from build123d import *

# Parameters (mm, degrees)
SKETCH1_W           = 38.1
SKETCH1_H           = 19.05
SKETCH1_R           = 3.175
SKETCH1_H_2         = 12.7
BOSS_EXTRUDE2_DEPTH = 12.7
SKETCH3_W           = 12.7
SKETCH3_H           = 31.75
SKETCH3_H_2         = 12.7
BOSS_EXTRUDE3_DEPTH = 38.1


with BuildPart() as part:
    # Sketch1 → Boss-Extrude2 (new body)
    # profile 1 of 3: a face of its own
    with BuildSketch(Plane(origin=(0, 0, 0), x_dir=(1, 0, 0), z_dir=(0, 1, 0))):
        Rectangle(SKETCH1_W, SKETCH1_H)
        with Locations(Location((0, 0, 0), (0, 0, 270))):
            Circle(SKETCH1_R, mode=Mode.SUBTRACT)
    # profile 2 of 3: a face of its own
    with BuildSketch(Plane(origin=(0, 0, 0), x_dir=(1, 0, 0), z_dir=(0, 1, 0))):
        with Locations((0, -15.875)):
            Rectangle(SKETCH1_W, SKETCH1_H_2)
    # profile 3 of 3: a face of its own
    with BuildSketch(Plane(origin=(0, 0, 0), x_dir=(1, 0, 0), z_dir=(0, 1, 0))):
        with Locations((0, -31.75)):
            Rectangle(SKETCH1_W, SKETCH1_H)
        with Locations(Location((0, -31.75, 0), (0, 0, 270))):
            Circle(SKETCH1_R, mode=Mode.SUBTRACT)
    extrude(amount=BOSS_EXTRUDE2_DEPTH)

    # Sketch3 → Boss-Extrude3 (add)
    with BuildSketch(Plane.XY.offset(34.925)):
        with BuildLine():
            ThreePointArc((-31.75, 31.75), (-38.1, 38.1), (-44.45, 31.75))
            Line((-44.45, 31.75), (-57.15, 31.75))
            ThreePointArc((-57.15, 31.75), (-38.1, 50.8), (-19.05, 31.75))
            Line((-19.05, 31.75), (-31.75, 31.75))
        make_face()
        with Locations((-25.4, 15.875)):
            Rectangle(SKETCH3_W, SKETCH3_H)
        with Locations((-50.8, 25.4)):
            Rectangle(SKETCH3_W, SKETCH3_H_2)
    extrude(amount=-BOSS_EXTRUDE3_DEPTH)


solid = part.part
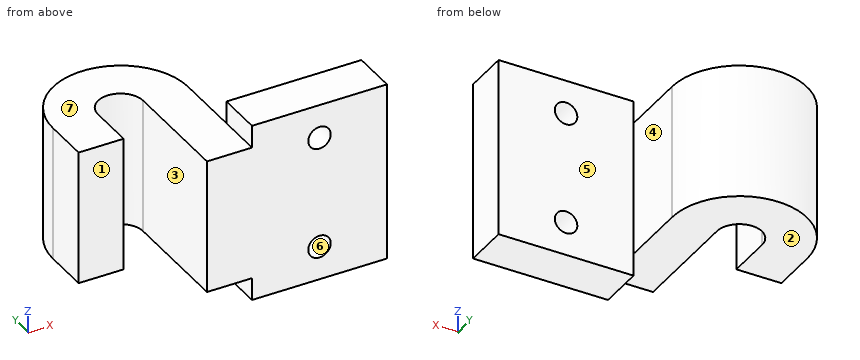
Geometry check sheet. Reference: the model listing, model coordinates, mm. Face numbers are marked on the shaded views. A direction names the side the tool comes from. Round coordinates to 2 decimals unless told otherwise and drop trailing zeros. Loops run counter-clockwise (first coordinate to the right, second up) from the corner with the lowest first, then second, coordinate; pieces in that order, holes last. Notation, with made-up numbers: (82.5, -4.75) - (133.5, -4.75) arc R23 ccw to (133.5, 18.25) - close; hole circle Ø1 at (-26.75, 80). An arc over 180 degrees is marked (long way). One line per question, with ' | ' between items. Start each with the question number.
1. Cross-section at A-A on x = 0. Record the cut outline in (y, z) (3 decimals), then the cut area to 3 significant figures.
2. Cross-section at D-D on y = 11. Record the cut outline in (x, z) (3 decimals), then the cut area to 3 significant figures.
3. Cross-section at B-B on y = 26.5. Record the cut outline in (x, z) (3 decimals), then the cut area to 3 significant figures.
4. Tool access check on the marked faces 1, 2, 3 and 4. Record the directions out of +Z, -Z, +X, -X, +Y, -Y that give a thin tool (end or side, any length) a straight path to the whole face; none if there is none.
5. Cross-section at C-C on z = 0. Record the cut outline in (x, y) (3 decimals).
6. Depth check by flat-ended pin: pin 1 (2 mm diameter, centred on x = 4.5, z = 21, fed in from +Y); pin 2 (6 mm diameter, centred on y = 11, z = -2.5, fed in from -X); pin 3 (8 mm diameter, centred on x = -25, z = 0, fed in from +Y); pin 4 (12 mm diameter, centred on x = 8, z = 30.5, fed in from -Y). Enter the tip coordinate at first touch or a pass-through.
7. Scan lines: line 1 (X direction, y = 28.5, z = 7); line 2 (X direction, y = 3, z = 0) (3 decimals); line 3 (Z direction, x = -21, y = 29.5) (3 decimals). Record each from-to range of solid material in increasing order. Write a range as [from, to].
8. Draft check along Z on the marked faces 5, 6 and 7. Enter one of: released by +Z, released by -Z, zero draft, split by the parting line, or undercut.
Taken from the geometry:
1) outline: (0, -9.525) - (12.7, -9.525) - (12.7, -3.175) - (0, -3.175) - close; (0, 3.175) - (12.7, 3.175) - (12.7, 28.575) - (0, 28.575) - close; (0, 34.925) - (12.7, 34.925) - (12.7, 41.275) - (0, 41.275) - close | area: 484 mm²
2) outline: (-31.75, -3.175) - (-19.05, -3.175) - (-19.05, -9.525) - (19.05, -9.525) - (19.05, 41.275) - (-19.05, 41.275) - (-19.05, 34.925) - (-31.75, 34.925) - close; hole circle Ø6.35 at (0, 0); hole circle Ø6.35 at (0, 31.75) | area: 2,360 mm²
3) outline: (-57.15, -3.175) - (-44.45, -3.175) - (-44.45, 34.925) - (-57.15, 34.925) - close; (-31.75, -3.175) - (-19.05, -3.175) - (-19.05, 34.925) - (-31.75, 34.925) - close | area: 968 mm²
4) face 1: +Z, -Z, -X, -Y | face 2: -Z, -X, +Y, -Y | face 3: +Z, -Z, -Y | face 4: +Z, -Z, +X, +Y
5) outline: (-57.15, 19.05) - (-44.45, 19.05) - (-44.45, 31.75) arc R6.35 cw to (-31.75, 31.75) - (-31.75, 0) - (-3.175, 0) - (-3.175, 12.7) - (-19.05, 12.7) - (-19.05, 31.75) arc R19.05 ccw to (-57.15, 31.75) - close; (3.175, 0) - (19.05, 0) - (19.05, 12.7) - (3.175, 12.7) - close
6) pin 1: y = 12.7 | pin 2: x = -31.75 | pin 3: y = 48.49 | pin 4: y = 0
7) line 1: [-57.15, -44.45], [-31.75, -19.05] | line 2: [-31.75, -3.175], [3.175, 19.05] | line 3: [-3.175, 34.925]
8) face 5: zero draft | face 6: undercut | face 7: released by +Z
